Verification items for the finished model (mm, model axes). Face numbers are marked on the shaded views. A direction names the side the tool comes from. Round coordinates to 2 decimals unless told otherwise and drop trailing zeros. Write each loop counter-clockwise with the first axis right and the second up, starting at its lowest first coordinate (ties: lowest second). Pieces come first, ordered by that corner, then holes. Notation, with made-up numbers: (-5, 32.25) -> (-1, 32.25) arc R25 cw to (-1, 64.25) -> close; hole circle Ø7 at (24, 66.25). An arc over 180 degrees is marked (long way). Answer as a JSON object with one key per item and string values. Group by question number.
(1) Sectioned sample at C-C on z = 12.75. Count the separate pieces of the cut face and the enclosed holes in it, and give its area (3 significant figures).
(2) Sectioned sample at A-A on y = 2.25. Record the cut outline in (x, z), and give its area (3 significant figures).
(3) Gauge pin test, flat ends, axial feed: pin 1 Ø1.6 at (x, z) = (-0.5, 12) entering from +Y; pin 2 Ø1.5 at (x, y) = (-0.5, 2) entering from -Z. Record the tip position at first contact, or that the pin passes through.
(4) Scan lines: L1, parallel to Y at x = 0, z = 14 (1 decimal); L2, parallel to X at y = 0.5, z = 12.75; L3, parallel to X at y = 6, z = 22. Record each from-to range of solid material in increasing order. Write a range as from..to.
(5) Draft check along X on the marked faces 1, 2 and 3. Enter one of: released by +X, released by -X, zero draft, split by the parting line, or undercut.
(6) Sectioned sample at B-B on x = 1. Record the cut outline in (y, z) (3 decimals), and give its area (3 significant figures).
(7) Sectioned sample at D-D on y = -5.75. Record the cut outline in (x, z).
(8) Set-up check for the marked faces 4 and 5: record each of +Z, -Z, +X, -X, +Y, -Y from which the full face is reachable in a straight line by a thin tool's end or side.
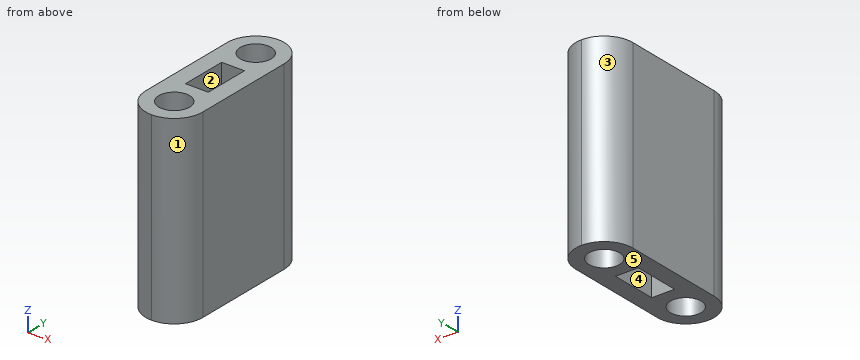
```python
from build123d import *

# Parameters (mm, degrees)
F0_W     = 7.9375
F0_H     = 22.225
F0_W_2   = 3.175
F0_H_2   = 6.35
F1_DEPTH = 25.4
F2_R     = 2.15265
F3_DEPTH = 25.4
F4_R     = 3.96874


# Not quite as in the source:
# - a fillet or chamfer is up to 0.001 mm smaller than in the source, because OpenCascade refuses the exact size


with BuildPart() as f1:
    # F0 (on Top) → F1 (new body)
    with BuildSketch(Plane.XY):
        Rectangle(F0_W, F0_H)
        Rectangle(F0_W_2, F0_H_2, mode=Mode.SUBTRACT)
    extrude(amount=F1_DEPTH)

    # F2 (on face) → F3 (cut, through all)
    with BuildSketch(Plane.XY.offset(25.4)):
        with Locations((0, 7.14375)):
            Circle(F2_R)
        with Locations((0, -7.14375)):
            Circle(F2_R)
    extrude(amount=-F3_DEPTH, mode=Mode.SUBTRACT)

    # F4 (radius 3.96875 in the source; OpenCascade refuses exactly that, so slightly less here)
    f4_edges = [f1.edges().sort_by_distance(p)[0] for p in [
        (-3.96875, -11.1125, 12.7),
        (3.96875, -11.1125, 12.7),
        (3.96875, 11.1125, 12.7),
        (-3.96875, 11.1125, 12.7),
    ]]
    fillet(f4_edges, radius=F4_R)


solid = f1.part
```
Computed values:
{
 "1": {"separate pieces": "1", "enclosed holes": "3", "area": "114 mm2"},
 "2": {"outline": "(-3.97, 0) -> (-1.59, 0) -> (-1.59, 25.4) -> (-3.97, 25.4) -> close; (1.59, 0) -> (3.97, 0) -> (3.97, 25.4) -> (1.59, 25.4) -> close", "area": "121 mm2"},
 "3": {"pin 1": "y = 11.11", "pin 2": "through"},
 "4": {"L1": "-11.1..-9.3, -5..-3.2, 3.2..5, 9.3..11.1", "L2": "-3.97..-1.59, 1.59..3.97", "L3": "-3.97..-1.82, 1.82..3.97"},
 "5": {"face 1": "released by +X", "face 2": "undercut", "face 3": "released by -X"},
 "6": {"outline": "(-10.984, 0) -> (-9.05, 0) -> (-9.05, 25.4) -> (-10.984, 25.4) -> close; (-5.237, 0) -> (-3.175, 0) -> (-3.175, 25.4) -> (-5.237, 25.4) -> close; (3.175, 0) -> (5.237, 0) -> (5.237, 25.4) -> (3.175, 25.4) -> close; (9.05, 0) -> (10.984, 0) -> (10.984, 25.4) -> (9.05, 25.4) -> close", "area": "203 mm2"},
 "7": {"outline": "(-3.97, 0) -> (-1.64, 0) -> (-1.64, 25.4) -> (-3.97, 25.4) -> close; (1.64, 0) -> (3.97, 0) -> (3.97, 25.4) -> (1.64, 25.4) -> close"},
 "8": {"face 4": "+Z, -Z", "face 5": "-Z, +X, -X, +Y, -Y"}
}
